Design review of the part built by this model. Coordinates are the model's own, in mm. Face numbers are marked on the shaded views. Coordinates: 2 decimals unless noted, no trailing zeros. Loops run counter-clockwise (first coordinate to the right, second up) from the corner with the lowest first, then second, coordinate; pieces in that order, holes last.
from build123d import *

# Parameters (mm, degrees)
SKETCH1_W            = 76.2
SKETCH1_H            = 50.8
BOSS_EXTRUDE2_DEPTH  = 2.54
SKETCH3_W            = 12.7
SKETCH3_H            = 10.16
BOSS_EXTRUDE3_DEPTH  = 0.254
LPATTERN2_COUNT      = 4
LPATTERN2_PITCH      = 17.78
LPATTERN2_COUNT_DIR2 = 3
LPATTERN2_PITCH_DIR2 = 15.24


with BuildPart() as part:
    # Sketch1 → Boss-Extrude2 (new body)
    with BuildSketch(Plane.XY):
        Rectangle(SKETCH1_W, SKETCH1_H)
    extrude(amount=BOSS_EXTRUDE2_DEPTH)

    # Sketch3 → Boss-Extrude3 (add)
    with BuildSketch(Plane.XY.offset(2.54)):
        with Locations((-26.67, 15.24)):
            Rectangle(SKETCH3_W, SKETCH3_H)
    boss_extrude3 = extrude(amount=BOSS_EXTRUDE3_DEPTH)

    # LPattern2: Boss-Extrude3 4 × 3
    with Locations(*[(i * LPATTERN2_PITCH, -j * LPATTERN2_PITCH_DIR2, 0) for i in range(LPATTERN2_COUNT) for j in range(LPATTERN2_COUNT_DIR2) if (i, j) != (0, 0)]):
        add(boss_extrude3)


solid = part.part
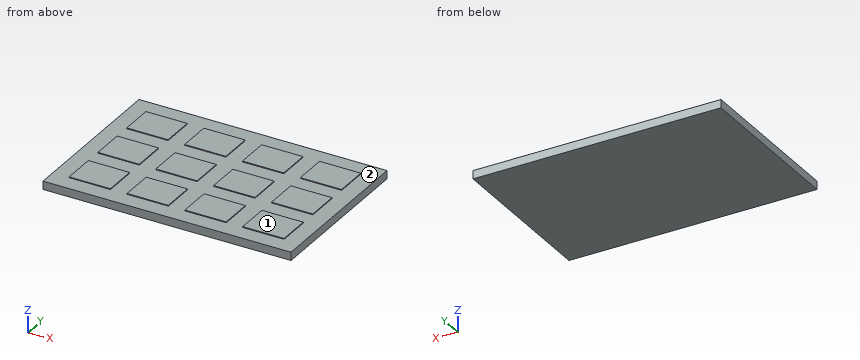
Q1. Take a section at B-B, the plane x = -7. Write out the cut boundary in (y, z).
Q2. Take a section at D-D, the plane y = 9. Write out the cut boundary in (x, z), then the cut area to 3 significant figures.
Q3. The part is to be moulded in two halves that separate along Y. For the marked faces 1 and 2, say which applies: pulls with the +Y half, pulls with the -Y half, needs draft (parallel to the pull), parting line crosses it, or undercut.
Q4. Take a section at A-A, the plane y = -11. Write out the cut boundary in (x, z).
Q5. Take a section at C-C, the plane x = 16.5. Write out the cut boundary in (y, z), then the cut area to 3 significant figures.
Q6. For line 1 (Y direction, x = -27, z = 2.65); line 2 (Z direction, x = 3.5, y = 7.5), list the stretches that pass through material, from the lowest coordinate up.
Entries:
1. outline: (-25.4, 0) - (25.4, 0) - (25.4, 2.54) - (20.32, 2.54) - (20.32, 2.79) - (10.16, 2.79) - (10.16, 2.54) - (5.08, 2.54) - (5.08, 2.79) - (-5.08, 2.79) - (-5.08, 2.54) - (-10.16, 2.54) - (-10.16, 2.79) - (-20.32, 2.79) - (-20.32, 2.54) - (-25.4, 2.54) - close
2. outline: (-38.1, 0) - (38.1, 0) - (38.1, 2.54) - (-38.1, 2.54) - close
2. area: 194 mm2
3. face 1: needs draft
3. face 2: undercut
4. outline: (-38.1, 0) - (38.1, 0) - (38.1, 2.54) - (33.02, 2.54) - (33.02, 2.79) - (20.32, 2.79) - (20.32, 2.54) - (15.24, 2.54) - (15.24, 2.79) - (2.54, 2.79) - (2.54, 2.54) - (-2.54, 2.54) - (-2.54, 2.79) - (-15.24, 2.79) - (-15.24, 2.54) - (-20.32, 2.54) - (-20.32, 2.79) - (-33.02, 2.79) - (-33.02, 2.54) - (-38.1, 2.54) - close
5. outline: (-25.4, 0) - (25.4, 0) - (25.4, 2.54) - (-25.4, 2.54) - close
5. area: 129 mm2
6. line 1: y = -20.32 to -10.16, -5.08 to 5.08, 10.16 to 20.32
6. line 2: z = 0 to 2.54
